Input: dimensioned drawing with shaded views. Units: mm. Origin: part minimum x, y, z. A direction names the side the tool comes from. Coordinates: 2 decimals unless noted, no trailing zeros. Order: outer loops, then holes, each group sorted by start corner. A loop starts at its lowest first (then second) coordinate and runs counter-clockwise, first axis right, second up.
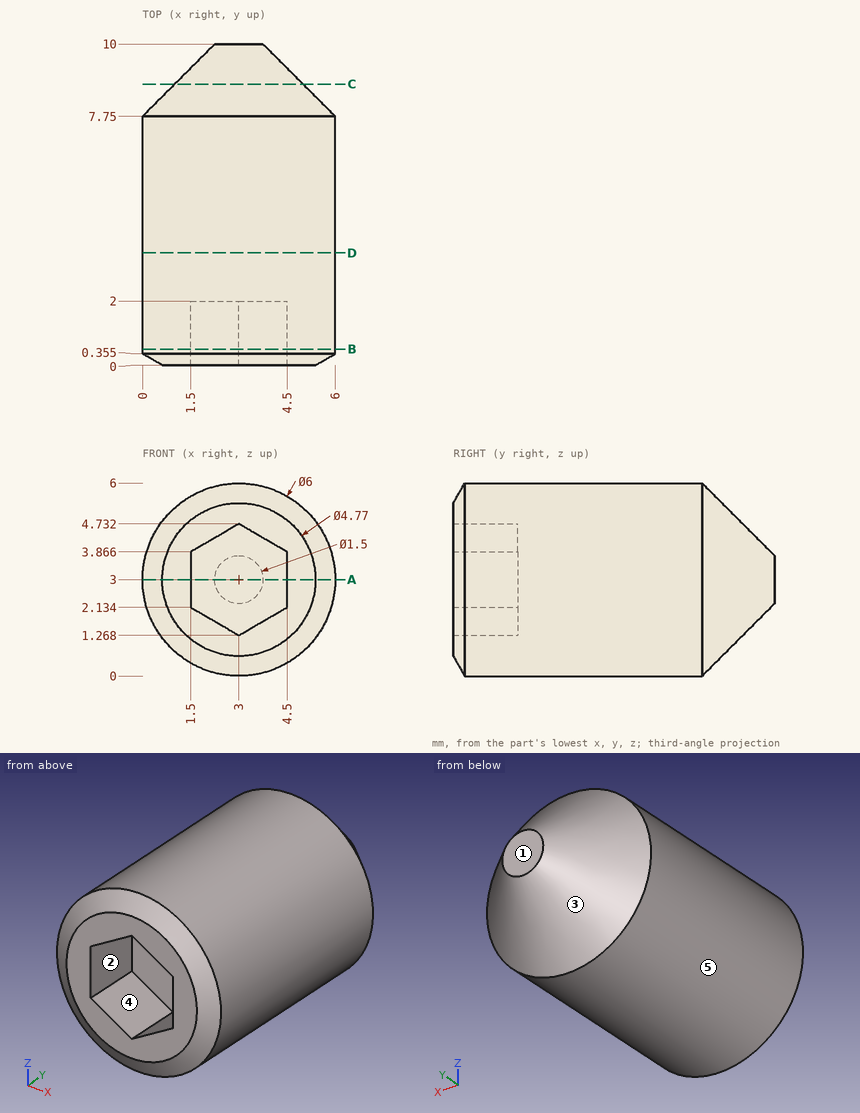
1. Ray query, line 1 (Z direction, x = 3.1, y = 7); line 2 (X direction, y = 1, z = 3.7); line 3 (Z direction, x = 4.3, y = 1.75). Return the intervals inside material, ascending.
Findings:
line 1: z = 0 to 6
line 2: x = 0.08 to 1.5, 4.5 to 5.92
line 3: z = 0.3 to 2.02, 3.98 to 5.7
2. Section query A-A on z = 3. Return loops of the section in (x, y) (3 decimals).
Findings:
outline: (0, 0.355) - (0.615, 0) - (1.5, 0) - (1.5, 2) - (4.5, 2) - (4.5, 0) - (5.385, 0) - (6, 0.355) - (6, 7.75) - (3.75, 10) - (2.25, 10) - (0, 7.75) - close
3. Access query for the marked faces 4 and 5. Directions: +Z, -Z, +X, -X, +Y, -Y. A direction counts if a zero-diameter tool reaches every point of the face in a straight line with its end or side. Return the directions, or none.
Findings:
face 4: -Y
face 5: +Y, -Y
4. Section query C-C on y = 8.75. Return loops of the section in (x, z).
Findings:
outline: circle Ø4 at (3, 3)
5. Section query B-B on y = 0.5. Return loops of the section in (x, z).
Findings:
outline: circle Ø6 at (3, 3); hole (1.5, 2.13) - (3, 1.27) - (4.5, 2.13) - (4.5, 3.87) - (3, 4.73) - (1.5, 3.87) - close
6. Section query D-D on y = 3.5. Return loops of the section in (x, z), plus the area to 3 significant figures.
Findings:
outline: circle Ø6 at (3, 3)
area: 28.3 mm2
7. Draft query along X for the marked faces 1, 2 and 3. Return one class per face: released by +X, released by -X, zero draft, split by the parting line, or undercut.
Findings:
face 1: zero draft
face 2: undercut
face 3: split by the parting line
